Can you work these out from the model? Positions are in its coordinate system, mm. A direction names the side the tool comes from. Round coordinates to 2 decimals unless told otherwise and drop trailing zeros. Write each loop counter-clockwise with the first axis right and the second up, starting at its lowest first coordinate (ties: lowest second). Pieces come first, ordered by that corner, then holes. Notation, with made-up numbers: (35, 15.25) -> (60, 15.25) arc R33 cw to (60, 54.25) -> close; hole circle Ø2 at (-3, 21). An arc over 180 degrees is marked (long way). Write item = value, one per line. Start each with the question number.
1) If I drill on line 1 (Y direction, x = 0, z = 7.75); line 2 (X direction, y = -10, z = 3.5); line 3 (Y direction, x = -12.5, z = 3.75), over which ranges is the centre line in solid material (lowest first)?
2) Thinking about a two-plate mould opening in Y: for faces 3 (the face through (-18, -18, 0)), 4 (the face through (-25.887, -4.351, 4.93)), 5 (the face through (23.091, -13.555, 4.93)), which applies, +Y half, -Y half, draft (parallel to the pull), parting line (faces both ways), or undercut?
3) Imagine slicing it at A-A, the plane x = 0. Please give me the cut outline in (y, z), then the cut area to 3 significant figures.
4) For faces 1 (the face through (-18, -18, 10)), 2 (the face through (9.175, 24.594, 4.93)), which set-ups out of +Z, -Z, +X, -X, +Y, -Y let a thin tool reach every point of the face, with its end or its side?
5) Imagine slicing it at B-B, the plane y = 3. Please give me the cut outline in (x, z), then the cut area to 3 significant figures.
6) I'm going to push flat-ended pins straight in: pin 1 (1 mm diameter, centred on x = -10.5, z = 4.5, fed in from +Y); pin 2 (1 mm diameter, centred on x = -18.5, z = 6, fed in from -Y); pin 3 (1 mm diameter, centred on y = 11.5, z = 2.5, fed in from -X). Where does each tip first touch, or does it pass through?
from build123d import *

# Parameters (mm, degrees)
CROQUIS1_R              = 25.25
SALIENTE_EXTRUIR1_DEPTH = 10


with BuildPart() as part:
    # Croquis1 → Saliente-Extruir1 (new body)
    with BuildSketch(Plane.XY):
        with BuildLine():
            Line((12.967631227, 22.823300382), (13.581702718, 23.555122287))
            Line((13.581702718, 23.555122287), (21.242147149, 17.12724619))
            Line((21.242147149, 17.12724619), (20.562408201, 16.317164857))
            ThreePointArc((20.562408201, 16.317164857), (22.866059206, 12.892084254), (24.60431654, 9.148229752))
            Line((24.60431654, 9.148229752), (25.545128646, 9.31412031))
            Line((25.545128646, 9.31412031), (27.281610423, -0.53395722))
            Line((27.281610423, -0.53395722), (26.240189935, -0.717587751))
            ThreePointArc((26.240189935, -0.717587751), (25.803289612, -4.822110037), (24.728368697, -8.807399251))
            Line((24.728368697, -8.807399251), (25.555704978, -9.285062076))
            Line((25.555704978, -9.285062076), (20.555704978, -17.945316114))
            Line((20.555704978, -17.945316114), (19.639895171, -17.416573075))
            ThreePointArc((19.639895171, -17.416573075), (16.666874037, -20.27998545), (13.281742316, -22.641948261))
            Line((13.281742316, -22.641948261), (13.608482931, -23.539660724))
            Line((13.608482931, -23.539660724), (4.211556723, -26.959862157))
            Line((4.211556723, -26.959862157), (3.849875184, -25.966150294))
            ThreePointArc((3.849875184, -25.966150294), (-0.268157132, -26.248630283), (-4.379558905, -25.882078042))
            Line((-4.379558905, -25.882078042), (-4.706299521, -26.779790505))
            Line((-4.706299521, -26.779790505), (-14.103225729, -23.359589072))
            Line((-14.103225729, -23.359589072), (-13.741544189, -22.365877208))
            ThreePointArc((-13.741544189, -22.365877208), (-17.077714598, -19.935249286), (-19.991615841, -17.01169586))
            Line((-19.991615841, -17.01169586), (-20.818952122, -17.489358685))
            Line((-20.818952122, -17.489358685), (-25.818952122, -8.829104647))
            Line((-25.818952122, -8.829104647), (-24.903142315, -8.300361608))
            ThreePointArc((-24.903142315, -8.300361608), (-25.896419606, -4.293943593), (-26.249373543, -0.181352121))
            Line((-26.249373543, -0.181352121), (-27.190185649, -0.015461563))
            Line((-27.190185649, -0.015461563), (-25.453703872, 9.832615967))
            Line((-25.453703872, 9.832615967), (-24.412283385, 9.648985436))
            ThreePointArc((-24.412283385, 9.648985436), (-22.597902074, 13.35654603), (-20.224757635, 16.733848291))
            Line((-20.224757635, 16.733848291), (-20.838829125, 17.465670196))
            Line((-20.838829125, 17.465670196), (-13.178384694, 23.893546292))
            Line((-13.178384694, 23.893546292), (-12.498645746, 23.083464959))
            ThreePointArc((-12.498645746, 23.083464959), (-8.725575014, 24.757359324), (-4.736752856, 25.819095112))
            Line((-4.736752856, 25.819095112), (-4.736752856, 26.774420761))
            Line((-4.736752856, 26.774420761), (5.263247144, 26.774420761))
            Line((5.263247144, 26.774420761), (5.263247144, 25.716934683))
            ThreePointArc((5.263247144, 25.716934683), (9.229545569, 24.573929042), (12.967631227, 22.823300382))
        make_face()
        Circle(CROQUIS1_R, mode=Mode.SUBTRACT)
    extrude(amount=SALIENTE_EXTRUIR1_DEPTH)


solid = part.part
Reported:
q1.line_1 = -26.25 to -25.25, 25.25 to 26.77
q1.line_2 = -25.14 to -23.19, 23.19 to 25.14
q1.line_3 = -23.94 to -21.94, 21.94 to 23.09
q2.face_3 = draft
q2.face_4 = undercut
q2.face_5 = -Y half
q3.outline = (-26.25, 0) -> (-25.25, 0) -> (-25.25, 10) -> (-26.25, 10) -> close; (25.25, 0) -> (26.77, 0) -> (26.77, 10) -> (25.25, 10) -> close
q3.area = 25.2 mm²
q4.face_1 = +Z, +X, -X, +Y, -Y
q4.face_2 = +Z, -Z, +Y
q5.outline = (-26.66, 0) -> (-25.07, 0) -> (-25.07, 10) -> (-26.66, 10) -> close; (25.07, 0) -> (26.66, 0) -> (26.66, 10) -> (25.07, 10) -> close
q5.area = 31.7 mm²
q6.pin_1 = 24.27
q6.pin_2 = -19.11
q6.pin_3 = -23.83
